Could you check a few things on this model? Use its own coordinates, in mm. A direction names the side the tool comes from. Give positions to 0.01 mm unless a question says otherwise; leave off trailing zeros. Loops run counter-clockwise (first coordinate to the right, second up) from the corner with the lowest first, then second, coordinate; pieces in that order, holes last. Notation, with made-up numbers: (6.25, 23) -> (15.25, 23) arc R22 cw to (15.25, 45) -> close; hole circle Ø7 at (79, -7.75). An arc over 180 degrees is marked (long way). Write each question's results on one line, items separated by ' | '. Start each with the question number.
Q1. If we section it at B-B, the plane y = -51: List the corners of the cut face in (x, z) for me, plus the area to 3 significant figures.
Q2. If we section it at A-A, the plane x = 96.5: List the corners of the cut face in (y, z) for me.
Q3. If we section it at C-C, the plane z = -40: List the corners of the cut face in (x, y) for me.
Q4. Which directions (+Z, -Z, +X, -X, +Y, -Y) give clear straight access to the entire face, cutting with the end or side of a thin tool? Please do faces 1 (the face through (-1.437, -64.4, -9.9)), 2 (the face through (76, -0.7, -59)).
Q5. If I drill on line 1 along X through (y, z) = (-31, -25.5); line 2 along Y through (x, z) = (98, -12.5), over which ranges is the centre line in solid material (lowest first)?
Q6. If we section it at D-D, the plane z = 38.5: List the corners of the cut face in (x, y) for me, plus the area to 3 significant figures.
Q7. Will these pins go through, and if not, where does the flat tip stop? P1, Ø0.6, axis at x = -1, z = 22.5, coming from the +Y side; P2, Ø0.8, axis at x = 106, y = -0.5, coming from the -Z side; P3, Ø2, axis at y = -78.5, z = -51.5, coming from the +X side.
from build123d import *

# Parameters (mm, degrees)
SKETCH1_W               = 125
SKETCH1_H               = 40
BASE_FLANGE1_DEPTH      = 0.7
CUT_EXTRUDE3_DEPTH      = 10
EDGE_FLANGE5_DEPTH      = 70
EDGE_FLANGE5_START      = 0.7
EDGE_FLANGE5_FLAT_DEPTH = 0.7
SKETCH26_W              = 0.7
SKETCH26_H              = 85
BOSS_EXTRUDE1_DEPTH     = 55
SKETCH27_W              = 0.7
SKETCH27_H              = 20
BOSS_EXTRUDE2_DEPTH     = 3
CUT_EXTRUDE4_START      = -63.5
CUT_EXTRUDE4_DEPTH      = 3.4
CUT_EXTRUDE4_START_2    = -1.4366
CUT_EXTRUDE4_2_DEPTH    = 0.7
SKETCH30_W              = 2.5
SKETCH30_H              = 19.2634
TAB1_DEPTH              = 0.7
BREAK_CORNER1_START     = -2
BREAK_CORNER1_DEPTH     = 2
BREAK_CORNER1_2_DEPTH   = 3
CUT_EXTRUDE5_DEPTH      = 7.5
SKETCH32_W              = 40
SKETCH32_H              = 32
CUT_EXTRUDE6_DEPTH      = 0.7
FILLET1_R               = 2.5


with BuildPart() as part:
    # Base-Flange1: sheet metal written as solids
    # Sketch1 → Base-Flange1 (new body)
    with BuildSketch(Plane(origin=(0, 0, 0), x_dir=(1, 0, 0), z_dir=(0, 1, 0))):
        Polygon((0, 0), (155, 0), (155, 70), (0, 70), (0, 55), (0, 15), align=None)
        with Locations((77.5, 35)):
            Rectangle(SKETCH1_W, SKETCH1_H, mode=Mode.SUBTRACT)
    extrude(amount=-BASE_FLANGE1_DEPTH)

    # Sketch22 → Cut-Extrude3 (cut)
    with BuildSketch(Plane(origin=(0, 0, 0), x_dir=(1, 0, 0), z_dir=(0, 1, 0))):
        with BuildLine():
            Line((10, 8.6), (148, 8.6))
            ThreePointArc((148, 8.6), (149.1, 7.5), (148, 6.4))
            Line((148, 6.4), (10, 6.4))
            ThreePointArc((10, 6.4), (8.9, 7.5), (10, 8.6))
        make_face()
    extrude(amount=-CUT_EXTRUDE3_DEPTH, mode=Mode.SUBTRACT)

    # Edge-Flange5: sheet metal written as solids
    # Edge-Flange5 bend section (on a plane across the edge) → Edge-Flange5 (add)
    with BuildSketch(Plane(origin=(-0.7366, -0.7, 0), x_dir=(1, 0, 0), z_dir=(0, 0, -1))):
        with BuildLine():
            Line((-0.7, 0.7366), (0, 0.7366))
            ThreePointArc((0, 0.7366), (0.215745145, 0.215745145), (0.7366, 0))
            Line((0.7366, 0), (0.7366, -0.7))
            ThreePointArc((0.7366, -0.7), (-0.279229602, -0.279229602), (-0.7, 0.7366))
        make_face()
    extrude(amount=EDGE_FLANGE5_DEPTH)

    # Edge-Flange5 profile (on flange) → Edge-Flange5 flat (add)
    with BuildSketch(Plane(origin=(-0.7366, -0.7, 0), x_dir=(0, 0, -1), z_dir=(-1, 0, 0)).offset(EDGE_FLANGE5_START)):
        Polygon((70, 0.7366), (70, 85), (55, 85), (55, 105), (0, 105), (0, 0.7366), align=None)
    extrude(amount=-EDGE_FLANGE5_FLAT_DEPTH)

    # Sketch26 → Boss-Extrude1 (add)
    with BuildSketch(Plane.XY):
        with Locations((-1.0866, -63.2)):
            Rectangle(SKETCH26_W, SKETCH26_H)
    extrude(amount=BOSS_EXTRUDE1_DEPTH)

    # Sketch27 → Boss-Extrude2 (add)
    with BuildSketch(Plane(origin=(0, 0, -70), x_dir=(-1, 0, 0), z_dir=(0, 0, -1))):
        with Locations((1.0866, -70.7)):
            Rectangle(SKETCH27_W, SKETCH27_H)
    extrude(amount=BOSS_EXTRUDE2_DEPTH)

    # Cut-Extrude4: read off the stored shape, not the designer's step
    # Cut-Extrude4 outline → Cut-Extrude4 (cut)
    with BuildSketch(Plane.XY.offset(CUT_EXTRUDE4_START)):
        with BuildLine():
            ThreePointArc((-0.7366, -1.4366), (-0.640617257, -1.073021825), (-0.377683113, -0.804195836))
            Line((-0.377683113, -0.804195836), (-0.7366, -0.203214415))
            ThreePointArc((-0.7366, -0.203214415), (-1.249403682, -0.727509033), (-1.4366, -1.4366))
            Line((-1.4366, -1.4366), (-1.4366, -20.7))
            Line((-1.4366, -20.7), (-0.7366, -20.7))
            Line((-0.7366, -20.7), (-0.7366, -1.4366))
        make_face()
    extrude(amount=CUT_EXTRUDE4_DEPTH, mode=Mode.SUBTRACT)

    # Cut-Extrude4 2 outline → Cut-Extrude4 2 (cut)
    with BuildSketch(Plane.YZ.offset(CUT_EXTRUDE4_START_2)):
        with BuildLine():
            Line((-20.7, -60.1), (-37.5, -60.1))
            ThreePointArc((-37.5, -60.1), (-39.2, -61.8), (-37.5, -63.5))
            Line((-37.5, -63.5), (-20.7, -63.5))
            Line((-20.7, -63.5), (-20.7, -60.1))
        make_face()
        with BuildLine():
            Line((-20.7, 48.5), (-37.5, 48.5))
            ThreePointArc((-37.5, 48.5), (-39.2, 46.8), (-37.5, 45.1))
            Line((-37.5, 45.1), (-20.7, 45.1))
            Line((-20.7, 45.1), (-20.7, 48.5))
        make_face()
    extrude(amount=CUT_EXTRUDE4_2_DEPTH, mode=Mode.SUBTRACT)

    # Tab1: sheet metal written as solids
    # Sketch30 → Tab1 (add)
    with BuildSketch(Plane.ZY.offset(1.4366)):
        with Locations((1.25, -11.0683)):
            Rectangle(SKETCH30_W, SKETCH30_H)
    extrude(amount=-TAB1_DEPTH)

    # Break-Corner1: read off the stored shape, not the designer's step
    # Break-Corner1 outline → Break-Corner1 (cut)
    with BuildSketch(Plane.YZ.offset(BREAK_CORNER1_START)):
        with BuildLine():
            Line((-105.7, 55), (-105.7, 52.5))
            ThreePointArc((-105.7, 52.5), (-104.967766953, 54.267766953), (-103.2, 55))
            Line((-103.2, 55), (-105.7, 55))
        make_face()
        with BuildLine():
            ThreePointArc((-60.7, -70.5), (-61.432233047, -72.267766953), (-63.2, -73))
            Line((-63.2, -73), (-60.7, -73))
            Line((-60.7, -73), (-60.7, -70.5))
        make_face()
        with BuildLine():
            ThreePointArc((-78.2, -73), (-79.967766953, -72.267766953), (-80.7, -70.5))
            Line((-80.7, -70.5), (-80.7, -73))
            Line((-80.7, -73), (-78.2, -73))
        make_face()
        with BuildLine():
            ThreePointArc((-83.2, -70), (-84.967766953, -69.267766953), (-85.7, -67.5))
            Line((-85.7, -67.5), (-85.7, -70))
            Line((-85.7, -70), (-83.2, -70))
        make_face()
        with BuildLine():
            ThreePointArc((-103.2, -55), (-104.967766953, -54.267766953), (-105.7, -52.5))
            Line((-105.7, -52.5), (-105.7, -55))
            Line((-105.7, -55), (-103.2, -55))
        make_face()
        with BuildLine():
            Line((-20.7, 48.5), (-20.7, 51))
            ThreePointArc((-20.7, 51), (-21.432233047, 49.232233047), (-23.2, 48.5))
            Line((-23.2, 48.5), (-20.7, 48.5))
        make_face()
        with BuildLine():
            Line((-20.7, 55), (-23.2, 55))
            ThreePointArc((-23.2, 55), (-21.432233047, 54.267766953), (-20.7, 52.5))
            Line((-20.7, 52.5), (-20.7, 55))
        make_face()
        with BuildLine():
            Line((-20.7, 45.1), (-23.2, 45.1))
            ThreePointArc((-23.2, 45.1), (-21.432233047, 44.367766953), (-20.7, 42.6))
            Line((-20.7, 42.6), (-20.7, 45.1))
        make_face()
        with BuildLine():
            Line((-1.4366, 2.5), (-3.9366, 2.5))
            ThreePointArc((-3.9366, 2.5), (-2.168833047, 1.767766953), (-1.4366, 0))
            Line((-1.4366, 0), (-1.4366, 2.5))
        make_face()
    extrude(amount=BREAK_CORNER1_DEPTH, mode=Mode.SUBTRACT)

    # Break-Corner1 2 outline → Break-Corner1 2 (cut)
    with BuildSketch(Plane(origin=(0, 0, 0), x_dir=(1, 0, 0), z_dir=(0, 1, 0)).offset(BREAK_CORNER1_START)):
        with BuildLine():
            Line((155, 0), (155, 2.5))
            ThreePointArc((155, 2.5), (154.267766953, 0.732233047), (152.5, 0))
            Line((152.5, 0), (155, 0))
        make_face()
        with BuildLine():
            ThreePointArc((152.5, 70), (154.267766953, 69.267766953), (155, 67.5))
            Line((155, 67.5), (155, 70))
            Line((155, 70), (152.5, 70))
        make_face()
    extrude(amount=BREAK_CORNER1_2_DEPTH, mode=Mode.SUBTRACT)

    # Sketch31 → Cut-Extrude5 (cut)
    with BuildSketch(Plane.ZY.offset(1.4366)):
        Polygon((-60.1, -5.420316857), (-63.5, -5.420316857), (-65.8, -1.4366), (-65.8, 0), (-57.8, 0), (-57.8, -1.4366), align=None)
    extrude(amount=-CUT_EXTRUDE5_DEPTH, mode=Mode.SUBTRACT)

    # Sketch32 → Cut-Extrude6 (cut)
    with BuildSketch(Plane.ZY.offset(1.4366)):
        with Locations((-30, -50)):
            Rectangle(SKETCH32_W, SKETCH32_H)
    extrude(amount=-CUT_EXTRUDE6_DEPTH, mode=Mode.SUBTRACT)

    # Fillet1
    fillet1_edges = [part.edges().sort_by_distance(p)[0] for p in [
        (15, -0.35, -55),
        (140, -0.35, -55),
        (140, -0.35, -15),
        (15, -0.35, -15),
        (6.0634, -0.35, -57.8),
        (6.0634, -0.35, -65.8),
        (-1.0866, -34, -10),
        (-1.0866, -66, -10),
        (-1.0866, -66, -50),
        (-1.0866, -34, -50),
    ]]
    fillet(fillet1_edges, radius=FILLET1_R)


solid = part.part
Final values:
1) outline: (-1.44, -70) -> (-0.74, -70) -> (-0.74, -50) -> (-1.44, -50) -> close; (-1.44, -10) -> (-0.74, -10) -> (-0.74, 55) -> (-1.44, 55) -> close | area: 59.5 mm²
2) outline: (-0.7, -70) -> (0, -70) -> (0, -55) -> (-0.7, -55) -> close; (-0.7, -15) -> (0, -15) -> (0, -8.6) -> (-0.7, -8.6) -> close; (-0.7, -6.4) -> (0, -6.4) -> (0, 0) -> (-0.7, 0) -> close
3) outline: (-1.44, -105.7) -> (-0.74, -105.7) -> (-0.74, -66) -> (-1.44, -66) -> close; (-1.44, -34) -> (-0.74, -34) -> (-0.74, -1.44) arc R0.74 cw to (0, -0.7) -> (15, -0.7) -> (15, 0) -> (0, 0) arc R1.44 ccw to (-1.44, -1.44) -> close; (140, -0.7) -> (155, -0.7) -> (155, 0) -> (140, 0) -> close
4) face 1: +Z, -Z, -X, +Y, -Y | face 2: +Z, -Z, +X, -Y
5) line 1: x = -1.44 to -0.74 | line 2: y = -0.7 to 0
6) outline: (-1.44, -105.7) -> (-0.74, -105.7) -> (-0.74, -20.7) -> (-1.44, -20.7) -> close | area: 59.5 mm²
7) P1: stops at y = -20.7 | P2: stops at z = -70 | P3: stops at x = -0.74
